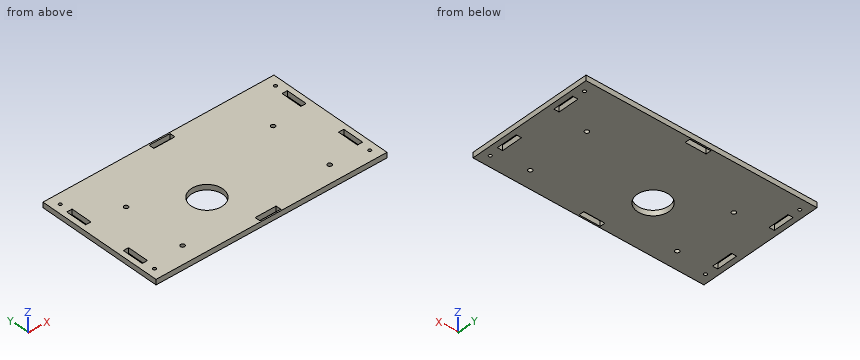
Autodesk Inventor part; units mm, degrees
ref_plane "YZ Plane" through (0, 0, 0) normal (1, 0, 0) x (0, 1, 0)
ref_plane "XZ Plane" through (0, 0, 0) normal (0, 1, 0) x (-1, 0, 0)
ref_plane "XY Plane" through (0, 0, 0) normal (0, 0, 1) x (1, 0, 0)
sketch "Sketch1" plane through (0, 0, 0) normal (0, 0, 1) x (1, 0, 0)
  circle A0 centre (1.016, 0) radius 19.05
  line L0 (159.5437, -28.575) -> (159.5437, 29.0493)
  line L1 (145.8277, 86.9876) -> (-55.3403, 86.9876)
  line L2 (159.5437, 93.3376) -> (-107.1563, 93.3376)
  line L3 (-107.1563, 93.3376) -> (-107.1563, -59.0624)
  line L4 (-107.1563, -59.0624) -> (159.5437, -59.0624)
  line L5 (159.5437, -59.0624) -> (159.5437, 93.3376)
  point P0 (0, 0)
  dimension "d0" = 266.7
  dimension "d1" = 152.4
  dimension "d15" = 38.1
extrude "Extrusion1" add sketch "Sketch1" along normal blind 6.35
sketch "Sketch2" plane through (0, 0, 6.35) normal (0, 0, 1) x (1, 0, 0)
  line L0 (-107.1563, 93.3376) -> (159.5437, 93.3376)
  line L1 (-107.1563, -59.0624) -> (-107.1563, 93.3376)
  line L2 (-103.9813, 93.3376) -> (-103.9813, -59.0624) construction
  circle A0 centre (-103.9813, 80.6376) radius 1.8542
  dimension "d4" = 3.175
  dimension "d5" = 3.7084
  dimension "d6" = 12.7
extrude "Extrusion2" cut sketch "Sketch2" against normal through all
pattern_linear "Rectangular Pattern1" count 2 spacing 127 along (0, -1, 0) count 2 spacing 260.35 along (1, 0, 0) of "Extrusion2"
sketch "Sketch3" plane through (0, 0, 0) normal (0, 0, -1) x (-1, 0, 0)
  circle A0 centre (62.484, 38.1) radius 2.5146
  circle A1 centre (62.484, -38.1) radius 2.5146
  circle A2 centre (-115.316, -38.1) radius 2.5146
  circle A3 centre (-115.316, 38.1) radius 2.5146
  point P0 (0, 0)
extrude "Extrusion3" cut sketch "Sketch3" against normal through all
sketch "Sketch4" plane through (0, 0, 0) normal (0, 0, -1) x (-1, 0, 0)
  line L0 (107.1563, 93.3376) -> (113.5063, 93.3376)
  line L1 (113.5063, 93.3376) -> (113.5063, -59.0624)
  line L2 (113.5063, -59.0624) -> (107.1563, -59.0624)
  line L3 (107.1563, -59.0624) -> (107.1563, 93.3376)
  line L4 (-159.5437, -59.0624) -> (-165.8937, -59.0624)
  line L5 (-165.8937, -59.0624) -> (-165.8937, 93.3376)
  line L6 (-165.8937, 93.3376) -> (-159.5437, 93.3376)
  line L7 (-159.5437, 93.3376) -> (-159.5437, -59.0624)
  point P0 (0, 0)
  dimension "d18" = 6.35
  dimension "d19" = 6.35
extrude "Extrusion4" add sketch "Sketch4" against normal blind 6.35
sketch "Sketch5" plane through (0, 0, 0) normal (0, 0, -1) x (-1, 0, 0)
  line L0 (-159.5437, -59.0624) -> (-159.5437, 93.3376)
  line L1 (-159.5437, 93.3376) -> (-153.1937, 93.3376)
  line L2 (-153.1937, -59.0624) -> (-153.1937, 93.3376)
  line L3 (-159.5437, -59.0624) -> (-153.1937, -59.0624)
  line L4 (-159.5437, 68.2942) -> (-153.1937, 68.2942)
  line L5 (-153.1937, 68.2942) -> (-153.1937, 42.8942)
  line L6 (-153.1937, 42.8942) -> (-159.5437, 42.8942)
  line L7 (-159.5437, 42.8942) -> (-159.5437, 68.2942)
  line L8 (-159.5437, -7.9058) -> (-153.1937, -7.9058)
  line L9 (-153.1937, -7.9058) -> (-153.1937, -33.3058)
  line L10 (-153.1937, -33.3058) -> (-159.5437, -33.3058)
  line L11 (-159.5437, -33.3058) -> (-159.5437, -7.9058)
  line L12 (100.8063, 68.2942) -> (107.1563, 68.2942)
  line L13 (107.1563, 68.2942) -> (107.1563, 42.8942)
  line L14 (107.1563, 42.8942) -> (100.8063, 42.8942)
  line L15 (100.8063, 42.8942) -> (100.8063, 68.2942)
  line L16 (100.8063, -7.9058) -> (107.1563, -7.9058)
  line L17 (107.1563, -7.9058) -> (107.1563, -33.3058)
  line L18 (107.1563, -33.3058) -> (100.8063, -33.3058)
  line L19 (100.8063, -33.3058) -> (100.8063, -7.9058)
  point P0 (0, 0)
  dimension "d22" = 25.4
  dimension "d25" = 76.2
  dimension "d28" = 260.35
extrude "Extrusion5" cut sketch "Sketch5" against normal through all contours L0 L8 L2 L10 | L0 L4 L2 L6 | L12 L13 L14 L15 | L16 L17 L18 L19
sketch "Sketch6" plane through (0, 0, 0) normal (0, 0, -1) x (-1, 0, 0)
  line L0 (-13.4937, 85.4001) -> (-13.4937, 91.7501)
  line L1 (-13.4937, 91.7501) -> (-38.8937, 91.7501)
  line L2 (-38.8937, 91.7501) -> (-38.8937, 85.4001)
  line L3 (-38.8937, 85.4001) -> (-13.4937, 85.4001)
  line L4 (-13.4937, -57.4749) -> (-13.4937, -51.1249)
  line L5 (-13.4937, -51.1249) -> (-38.8937, -51.1249)
  line L6 (-38.8937, -51.1249) -> (-38.8937, -57.4749)
  line L7 (-38.8937, -57.4749) -> (-13.4937, -57.4749)
  point P0 (0, 0)
extrude "Extrusion6" cut sketch "Sketch6" against normal through all
properties part number "panStepperMountRB02" material "Wood (Oak)"
Work out the finished part from the listing and answer in its coordinate system (mm). Coordinates: 2 decimals unless noted, no trailing zeros. Order: outer loops, then holes, each group sorted by start corner. A loop starts at its lowest first (then second) coordinate and runs counter-clockwise, first axis right, second up. Notation, with made-up numbers: (27, -35) - (48, -35) arc R20 ccw to (48, -26) - close; hole circle Ø10 at (25, 39). An arc over 180 degrees is marked (long way). Answer as a JSON object with one key per item and string values.
1. Find section D-D on z = 4.75. Count the separate pieces of the cut face and the enclosed holes in it, plus the area to 4 significant figures.
Output values:
{"separate pieces": "1", "enclosed holes": "15", "area": "40,350 mm²"}
2. Consider line 1 (X direction, y = 61.5, z = 1.25); line 2 (Y direction, x = 23, z = 5); line 3 (X direction, y = 80.5, z = 4.25). Determine where each line is inside the solid, lowest interval first.
Output values:
{"line 1": "x = -113.51 to -107.16, -100.81 to 153.19, 159.54 to 165.89", "line 2": "y = -59.06 to -57.47, -51.12 to 85.4, 91.75 to 93.34", "line 3": "x = -113.51 to -105.83, -102.13 to 154.52, 158.22 to 165.89"}
3. Find section C-C on y = 64.5. Determine the outline of the cut face in (x, z).
Output values:
{"outline": "(-113.51, 0) - (-107.16, 0) - (-107.16, 6.35) - (-113.51, 6.35) - close; (-100.81, 0) - (153.19, 0) - (153.19, 6.35) - (-100.81, 6.35) - close; (159.54, 0) - (165.89, 0) - (165.89, 6.35) - (159.54, 6.35) - close"}
4. Find section A-A on x = 33. Determine the outline of the cut face in (y, z), plus the area to 3 significant figures.
Output values:
{"outline": "(-59.06, 0) - (-57.47, 0) - (-57.47, 6.35) - (-59.06, 6.35) - close; (-51.12, 0) - (85.4, 0) - (85.4, 6.35) - (-51.12, 6.35) - close; (91.75, 0) - (93.34, 0) - (93.34, 6.35) - (91.75, 6.35) - close", "area": "887 mm²"}
5. Find section B-B on y = 0. Determine the outline of the cut face in (x, z).
Output values:
{"outline": "(-113.51, 0) - (-18.03, 0) - (-18.03, 6.35) - (-113.51, 6.35) - close; (20.07, 0) - (165.89, 0) - (165.89, 6.35) - (20.07, 6.35) - close"}
